Geometry: final body of the model. Coordinates: model frame, mm. Face numbers are marked on the shaded views. A direction names the side the tool comes from. Round coordinates to 2 decimals unless told otherwise and drop trailing zeros. Loops run counter-clockwise (first coordinate to the right, second up) from the corner with the lowest first, then second, coordinate; pieces in that order, holes last. Notation, with made-up numbers: M 31.5,-38.5 L 87.5,-38.5 A33 cw 87.5,-8.5 Z; hole C -30,33 d5. An arc over 180 degrees is marked long. Answer as a JSON object with one key per item and string values.
Autodesk Inventor part; units mm, degrees
ref_plane "YZ Plane" through (0, 0, 0) normal (1, 0, 0) x (0, 1, 0)
ref_plane "XZ Plane" through (0, 0, 0) normal (0, 1, 0) x (-1, 0, 0)
ref_plane "XY Plane" through (0, 0, 0) normal (0, 0, 1) x (1, 0, 0)
sketch "Sketch1" plane through (0, 0, 0) normal (0, 0, 1) x (1, 0, 0)
  line L0 (1.0583, 9.7858) -> (20.2702, 2.9934)
  line L1 (20.2702, -2.9934) -> (1.0583, -9.7858)
  line L2 (-1.0583, -9.7858) -> (-20.2702, -2.9934)
  line L3 (-20.2702, 2.9934) -> (-1.0583, 9.7858)
  arc A0 (20.2702, -2.9934) -> (20.2702, 2.9934) centre (19.2118, 0) ccw
  arc A1 (-20.2702, 2.9934) -> (-20.2702, -2.9934) centre (-19.2118, 0) ccw
  arc A2 (1.0583, 9.7858) -> (-1.0583, 9.7858) centre (0, 6.7924) ccw
  arc A3 (-1.0583, -9.7858) -> (1.0583, -9.7858) centre (0, -6.7924) ccw
  point P0 (0, 10.16)
  point P1 (28.7368, 0)
  point P2 (0, -10.16)
  point P3 (-28.7368, 0)
  point P4 (0, 0)
  dimension "d0" = 30.48
  dimension "d1" = 20.32
  dimension "d2" = 3.175
extrude "Extrusion1" add sketch "Sketch1" along normal blind 6.35
sketch "Sketch2" plane through (0, 0, 6.35) normal (0, 0, 1) x (1, 0, 0)
  circle A0 centre (0, 0) radius 4.4138
extrude "Extrusion2" cut sketch "Sketch2" against normal blind 2.54
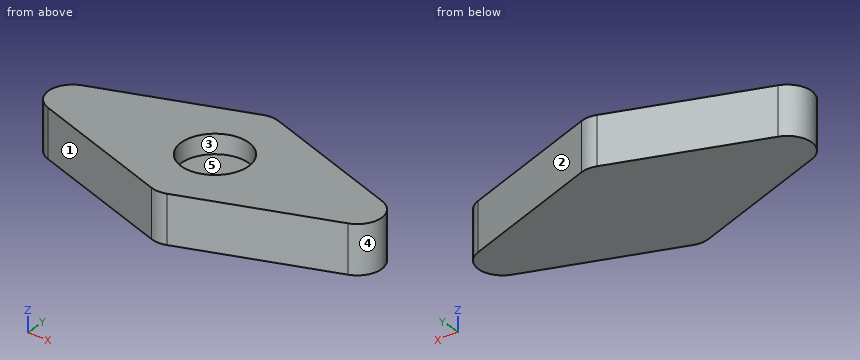
1) Set-up query: the marked faces 4 and 5. Return all of +Z, -Z, +X, -X, +Y, -Y with unobstructed straight access to the full face (end or side cutting, diameter ignored); none if empty.
Geometry results:
{"face 4": "+Z, -Z, +X", "face 5": "+Z"}
2) Pull-direction query (X, two-part tool) for the marked faces 1, 2 and 3; classes: +X half, -X half, draft (parallel to the pull), parting line (faces both ways), or undercut.
Geometry results:
{"face 1": "-X half", "face 2": "+X half", "face 3": "undercut"}
3) Cut plane A-A on z = 5. Return the cut outline in (x, y) (3 decimals).
Geometry results:
{"outline": "M -20.27,-2.993 L -1.058,-9.786 A3.175 ccw 1.058,-9.786 L 20.27,-2.993 A3.175 ccw 20.27,2.993 L 1.058,9.786 A3.175 ccw -1.058,9.786 L -20.27,2.993 A3.175 ccw Z; hole C 0,0 d8.828"}
4) Cut plane D-D on y = -8.5. Return the cut outline in (x, z), and give its area (3 significant figures).
Geometry results:
{"outline": "M -4.7,0 L 4.7,0 L 4.7,6.35 L -4.7,6.35 Z", "area": "59.6 mm2"}
5) First-contact query: pin 1 (4 mm diameter, centred on x = 15, y = -5.5, fed in from -Z); pin 2 (2.5 mm diameter, centred on x = 0, y = 0.5, fed in from +Z); pin 3 (1.5 mm diameter, centred on x = 5.5, z = 2, fed in from +Y). Flat tips, straight axial feed; report the tip coordinate or a pass-through.
Geometry results:
{"pin 1": "z = 0", "pin 2": "z = 3.81", "pin 3": "y = 8.48"}
6) Cut plane C-C on z = 2.75. Return the cut outline in (x, y) (3 decimals).
Geometry results:
{"outline": "M -20.27,-2.993 L -1.058,-9.786 A3.175 ccw 1.058,-9.786 L 20.27,-2.993 A3.175 ccw 20.27,2.993 L 1.058,9.786 A3.175 ccw -1.058,9.786 L -20.27,2.993 A3.175 ccw Z"}
7) Cut plane B-B on x = 0. Return the cut outline in (y, z), and give its area (3 significant figures).
Geometry results:
{"outline": "M -9.97,0 L 9.97,0 L 9.97,6.35 L 4.41,6.35 L 4.41,3.81 L -4.41,3.81 L -4.41,6.35 L -9.97,6.35 Z", "area": "104 mm2"}
8) Line query: probe 1 along Y at (x, z) = (0, 4.75); probe 2 along Y at (x, z) = (-3, 5.25); probe 3 along Z at (x, y) = (-1, 2.25). Output: solid intervals per line, ascending.
Geometry results:
{"probe 1": "-9.97 to -4.41, 4.41 to 9.97", "probe 2": "-9.1 to -3.24, 3.24 to 9.1", "probe 3": "0 to 3.81"}
